Geometry: final body of the model. Coordinates: model frame, mm. A direction names the side the tool comes from. Coordinates: 2 decimals unless noted, no trailing zeros. Order: outer loops, then holes, each group sorted by start corner. A loop starts at its lowest first (then second) coordinate and runs counter-clockwise, first axis right, second up. Notation, with made-up numbers: (80.5, 84) -> (117.5, 84) arc R38 ccw to (117.5, 122) -> close; hole circle Ø5 at (62.5, -7). An arc over 180 degrees is marked (long way). Use one line per item in the form item = value.
```python
from build123d import *

# Parameters (mm, degrees)
SKETCH1_R           = 17.25
SKETCH1_R_2         = 9.5
BOSS_EXTRUDE1_DEPTH = 20
CUT_EXTRUDE1_START  = -15.5
SKETCH2_R           = 17.25
SKETCH2_R_2         = 14.5
CUT_EXTRUDE1_DEPTH  = 15.5
CHAMFER1_SIZE       = 1


with BuildPart() as part:
    # Sketch1 → Boss-Extrude1 (new body)
    with BuildSketch(Plane(origin=(0, 0, 0), x_dir=(1, 0, 0), z_dir=(0, 1, 0))):
        with Locations(Location((0, 0, 0), (0, 0, 270))):
            Circle(SKETCH1_R)
        with Locations(Location((0, 0, 0), (0, 0, 270))):
            Circle(SKETCH1_R_2, mode=Mode.SUBTRACT)
    extrude(amount=BOSS_EXTRUDE1_DEPTH)

    # Sketch2 → Cut-Extrude1 (cut)
    with BuildSketch(Plane(origin=(0, 20, 0), x_dir=(1, 0, 0), z_dir=(0, 1, 0)).offset(CUT_EXTRUDE1_START)):
        with Locations(Location((0, 0, 0), (0, 0, 270))):
            Circle(SKETCH2_R)
        with Locations(Location((0, 0, 0), (0, 0, 270))):
            Circle(SKETCH2_R_2, mode=Mode.SUBTRACT)
    extrude(amount=CUT_EXTRUDE1_DEPTH, mode=Mode.SUBTRACT)

    # Chamfer1
    chamfer1_edges = [part.edges().sort_by_distance(p)[0] for p in [
        (0, 20, -14.5),
    ]]
    chamfer(chamfer1_edges, length=CHAMFER1_SIZE)


solid = part.part
```
1) Contact query for flat-ended pins moving along their axis: P1, Ø3, axis at y = 8, z = 11.5, coming from the +X side; P2, Ø10, axis at y = 8.5, z = 2, coming from the +X side; P3, Ø4, axis at x = 3, y = 12, coming from the +Z side; P4, Ø5, axis at x = -11.5, y = 10, coming from the +Z side. Output: stop coordinate, or through.
Results found:
P1 = 10.5
P2 = 17.25
P3 = 14.47
P4 = 11.37
2) Pull-direction query (Z, two-part tool) for faces 3 (the cylindrical face through (-5.78, 9.86, -7.54)), 4 (the flat face through (9.2, 20, -3.2)), 5 (the cylindrical face through (-5.554, 11.648, 13.394)); classes: released by +Z, released by -Z, zero draft, split by the parting line, or undercut.
Results found:
face_3 = undercut
face_4 = zero draft
face_5 = split by the parting line
3) Material intervals for probe 1 along X at (y, z) = (9, 0); probe 2 along X at (y, z) = (4, 0); probe 3 along Z at (x, y) = (4, 4.25), sorted ascending. Write a range as from..to.
Results found:
probe_1 = -14.5..-9.5, 9.5..14.5
probe_2 = -17.25..-9.5, 9.5..17.25
probe_3 = -16.78..-8.62, 8.62..16.78
4) Section C-C, the plane y = 7.75. Output: boundary loops of the cut face in (x, z).
Results found:
outline = circle Ø29 at (0, 0); hole circle Ø19 at (0, 0)
5) Section B-B, the plane y = 3.25. Output: boundary loops of the cut face in (x, z).
Results found:
outline = circle Ø34.5 at (0, 0); hole circle Ø19 at (0, 0)
6) Access query for faces 1 (the cylindrical face through (0.758, 2.218, -17.233)), 2 (the flat face through (14.14, 4.5, -3.91)). Directions: +Z, -Z, +X, -X, +Y, -Y. A direction counts if a zero-diameter tool reaches every point of the face in a straight line with its end or side. Return the directions, or none.
Results found:
face_1 = +Y, -Y
face_2 = +Y
7) Section A-A, the plane z = 0. Output: boundary loops of the cut face in (x, y).
Results found:
outline = (-17.25, 0) -> (-9.5, 0) -> (-9.5, 20) -> (-13.5, 20) -> (-14.5, 19) -> (-14.5, 4.5) -> (-17.25, 4.5) -> close; (9.5, 0) -> (17.25, 0) -> (17.25, 4.5) -> (14.5, 4.5) -> (14.5, 19) -> (13.5, 20) -> (9.5, 20) -> close
